Here's the drawing with two shaded views (mm, measured from the low corner). I have some questions. Give positions to 0.01 mm unless a question says otherwise; leave off trailing zeros. Order: outer loops, then holes, each group sorted by start corner. A loop starts at its lowest first (then second) coordinate and runs counter-clockwise, first axis right, second up. Notation, with made-up numbers: M 56,48 L 60,48 A19 cw 60,61 Z; hole C -9,12 d11. An arc over 180 degrees is marked long. One line per question, with ' | ' between items. Start each with the question number.
1) Please list where these lines run through material, in increasing order: line 1 along X through (y, z) = (59.5, 0.5); line 2 along Y through (x, z) = (167, 3.75); line 3 along Y through (x, z) = (184.5, 5.25). Write a range as [from, to].
2) If we section it at B-B, the plane y = 148.5: Please give me the cut outline in (x, z).
3) If we section it at C-C, the plane z = 5.25: Please give me the cut outline in (x, y), plus the area to 3 significant figures.
4) If we section it at A-A, the plane x = 114: Please give me the cut outline in (y, z).
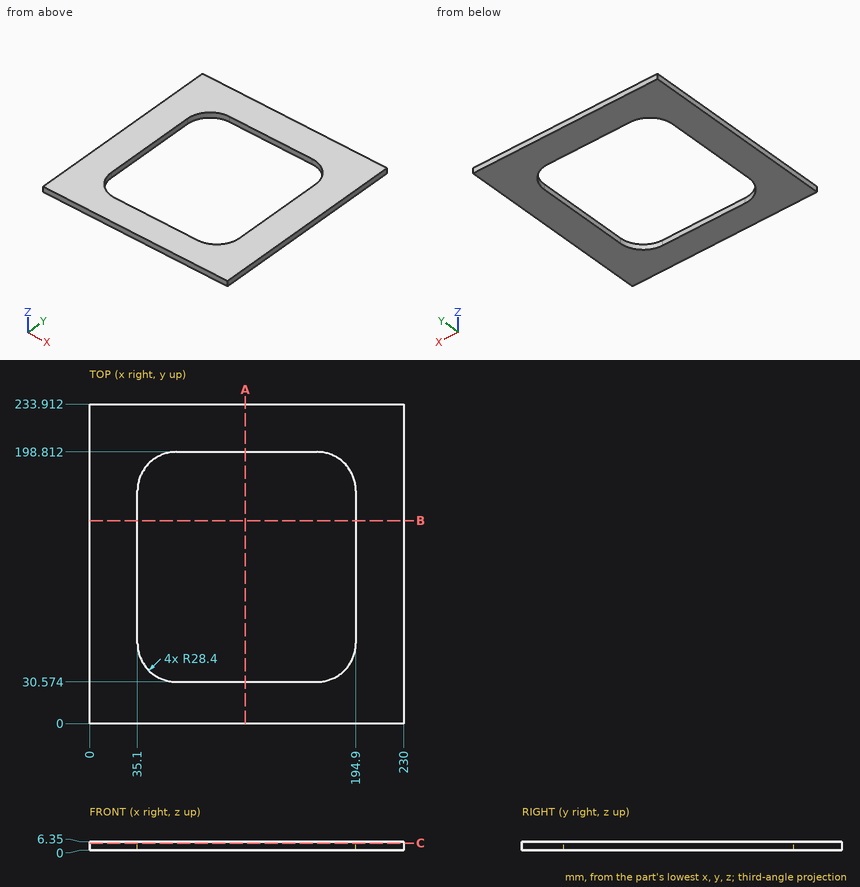
Results found:
1) line 1: x = [0, 35.1], [194.9, 230] | line 2: y = [0, 30.58], [198.81, 233.91] | line 3: y = [0, 37.01], [192.38, 233.91]
2) outline: M 0,0 L 35.1,0 L 35.1,6.35 L 0,6.35 Z; M 194.9,0 L 230,0 L 230,6.35 L 194.9,6.35 Z
3) outline: M 0,0 L 230,0 L 230,233.91 L 0,233.91 Z; hole M 35.1,58.97 A28.4 ccw 63.5,30.57 L 166.5,30.57 A28.4 ccw 194.9,58.97 L 194.9,170.41 A28.4 ccw 166.5,198.81 L 63.5,198.81 A28.4 ccw 35.1,170.41 Z | area: 27,600 mm²
4) outline: M 0,0 L 30.57,0 L 30.57,6.35 L 0,6.35 Z; M 198.81,0 L 233.91,0 L 233.91,6.35 L 198.81,6.35 Z
